from build123d import *

# Parameters (mm, degrees)
ESQUISSE1_R             = 1.5
BOSS_EXTRU_1_DEPTH      = 6
ESQUISSE2_R             = 1.5
ENL_V_MAT_EXTRU_1_DEPTH = 28.676885663
ESQUISSE3_R             = 1.5
ENL_V_MAT_EXTRU_2_DEPTH = 22.90010149


with BuildPart() as part:
    # Esquisse1 → Boss.-Extru.1 (new body)
    with BuildSketch(Plane.XY):
        with BuildLine():
            Line((-10, 4.424421769), (-10, -4.424421769))
            ThreePointArc((-10, -4.424421769), (-9.671289073, -5.165617412), (-8.901258038, -5.41953484))
            ThreePointArc((-8.901258038, -5.41953484), (-6.517555279, -6.205559881), (-5.5, -8.5))
            Line((-5.5, -8.5), (-5.5, -11.715481211))
            ThreePointArc((-5.5, -11.715481211), (-5.324186186, -12.281800142), (-4.858565737, -12.64898569))
            ThreePointArc((-4.858565737, -12.64898569), (0, -13.55), (4.858565737, -12.64898569))
            ThreePointArc((4.858565737, -12.64898569), (5.324186186, -12.281800142), (5.5, -11.715481211))
            Line((5.5, -11.715481211), (5.5, 1.096471453))
            ThreePointArc((5.5, 1.096471453), (5.66862168, 1.65217829), (6.117620177, 2.020476687))
            ThreePointArc((6.117620177, 2.020476687), (8.124885753, 5.023493695), (6.117620177, 8.026510703))
            ThreePointArc((6.117620177, 8.026510703), (5.66862168, 8.394809099), (5.5, 8.950515936))
            Line((5.5, 8.950515936), (5.5, 11.715481211))
            ThreePointArc((5.5, 11.715481211), (5.324186186, 12.281800142), (4.858565737, 12.64898569))
            ThreePointArc((4.858565737, 12.64898569), (0, 13.55), (-4.858565737, 12.64898569))
            ThreePointArc((-4.858565737, 12.64898569), (-5.324186186, 12.281800142), (-5.5, 11.715481211))
            Line((-5.5, 11.715481211), (-5.5, 8.5))
            ThreePointArc((-5.5, 8.5), (-6.517555279, 6.205559881), (-8.901258038, 5.41953484))
            ThreePointArc((-8.901258038, 5.41953484), (-9.671289073, 5.165617412), (-10, 4.424421769))
        make_face()
        with Locations((-4.874885753, -5.023493695)):
            Circle(ESQUISSE1_R, mode=Mode.SUBTRACT)
        with Locations((4.874885753, 5.023493695)):
            Circle(ESQUISSE1_R, mode=Mode.SUBTRACT)
        with BuildLine():
            Line((-3.5, 11.55), (3.5, 11.55))
            Line((3.5, 11.55), (3.5, 8.5))
            ThreePointArc((3.5, 8.5), (0, 5), (-3.5, 8.5))
            Line((-3.5, 8.5), (-3.5, 11.55))
        make_face(mode=Mode.SUBTRACT)
        with BuildLine():
            Line((-3.5, -11.55), (3.5, -11.55))
            Line((3.5, -11.55), (3.5, -8.5))
            ThreePointArc((3.5, -8.5), (0, -5), (-3.5, -8.5))
            Line((-3.5, -8.5), (-3.5, -11.55))
        make_face(mode=Mode.SUBTRACT)
        with BuildLine():
            Line((0, -3), (-8, -3))
            Line((-8, -3), (-8, 3))
            Line((-8, 3), (0, 3))
            ThreePointArc((0, 3), (3, 0), (0, -3))
        make_face(mode=Mode.SUBTRACT)
    extrude(amount=BOSS_EXTRU_1_DEPTH)

    # Esquisse2 → Enlèv. mat.-Extru.1 (cut, through all)
    with BuildSketch(Plane.XZ.offset(-11.55)):
        with Locations(Location((0, 3, 0), (0, 0, 270))):
            Circle(ESQUISSE2_R)
    enl_v_mat_extru_1 = extrude(amount=-ENL_V_MAT_EXTRU_1_DEPTH, mode=Mode.SUBTRACT)

    # Symétrie1: Enlèv. mat.-Extru.1 across plane
    add(enl_v_mat_extru_1.mirror(Plane.ZX), mode=Mode.SUBTRACT)

    # Esquisse3 → Enlèv. mat.-Extru.2 (cut, through all)
    with BuildSketch(Plane(origin=(-8, 0, 0), x_dir=(0, 0, -1), z_dir=(1, 0, 0))):
        with Locations((-3, 0)):
            Circle(ESQUISSE3_R)
    extrude(amount=-ENL_V_MAT_EXTRU_2_DEPTH, mode=Mode.SUBTRACT)


solid = part.part
For this review, take the finished solid that the model builds, in its own axes (mm). A direction names the side the tool comes from. Give positions to 0.01 mm unless a question says otherwise; leave off trailing zeros. Order: outer loops, then holes, each group sorted by start corner. A loop starts at its lowest first (then second) coordinate and runs counter-clockwise, first axis right, second up. Notation, with made-up numbers: (17.5, 2) - (64.5, 2) arc R25 ccw to (64.5, 38) - close; hole circle Ø9 at (87.25, -14.5). An arc over 180 degrees is marked (long way). Answer as a JSON object with one key per item and string values. Group by question number.
Item 1: Take a section at C-C on x = -2. Give the boundary of the cut face in (y, z).
Item 2: Wall thickness on line 1 along Y through (x, z) = (0, 2.5); line 2 along Y through (x, z) = (-5.25, 0.5); line 3 along Z through (x, y) = (0, -12.6): over which ranges is each line inside the solid? List them lowest first.
Item 3: Take a section at A-A on y = 0. Give the boundary of the cut face in (x, z).
Item 4: Take a section at D-D on x = -7.5. Give the boundary of the cut face in (y, z).
Item 5: Take a section at B-B on x = -4.25. Give the boundary of the cut face in (y, z).
Item 6: Machinability: for faces 4 (the flat face through (5.5, 10, 3)), 5 (the cylindrical face through (-8.99, 0.45, 1.57)), 6 (the flat face through (3.5, -10, 3)), 7 (the flat face through (-5.5, 10, 3)), which of the approach directions +Z, -Z, +X, -X, +Y, -Y give a long, thin tool a straight path to every point of the face, cutting with its end or side? Answer none if there is none.
Item 7: Draft analysis for pull direction X (two halves, no side actions). For faces 1 (the flat face through (-3.5, -10, 3)), 2 (the cylindrical face through (1.17, 13.5, 1.62)), 3 (the flat face through (-5.5, -10, 3)), state which applies: pulls with the +X half, pulls with the -X half, needs draft (parallel to the pull), parting line crosses it, or undercut.
Item 8: Clearance check with flat-ended pins moving along their axes: pin 1 Ø2.5 at (y, z) = (0, 3) entering from +X; pin 2 Ø2.5 at (x, y) = (-4.87, -5.02) entering from +Z; pin 3 Ø3.5 at (y, z) = (-9.5, 1.5) entering from -X; pin 4 Ø2.5 at (x, z) = (0, 3) entering from -Y. State where each tip first meets the part, or that it passes through.
Reported:
{
 "1": {"outline": "(-13.4, 0) - (-11.55, 0) - (-11.55, 6) - (-13.4, 6) - close; (-5.63, 0) - (-3, 0) - (-3, 6) - (-5.63, 6) - close; (3, 0) - (5.63, 0) - (5.63, 6) - (3, 6) - close; (11.55, 0) - (13.4, 0) - (13.4, 6) - (11.55, 6) - close"},
 "2": {"line 1": "-5 to -3, 3 to 5", "line 2": "-12.38 to -6.48, -3.57 to -3, 3 to 12.38", "line 3": "0 to 1.5, 4.5 to 6"},
 "3": {"outline": "(-10, 0) - (-8, 0) - (-8, 1.5) - (-10, 1.5) - close; (-10, 4.5) - (-8, 4.5) - (-8, 6) - (-10, 6) - close; (3, 0) - (5.5, 0) - (5.5, 6) - (3, 6) - close"},
 "4": {"outline": "(-5.6, 0) - (-3, 0) - (-3, 6) - (-5.6, 6) - close; (3, 0) - (5.6, 0) - (5.6, 6) - (3, 6) - close"},
 "5": {"outline": "(-12.87, 0) - (-6.39, 0) - (-6.39, 6) - (-12.87, 6) - close; (-3.66, 0) - (-3, 0) - (-3, 6) - (-3.66, 6) - close; (3, 0) - (12.87, 0) - (12.87, 6) - (3, 6) - close"},
 "6": {"face 4": "+Z, -Z, +X, +Y", "face 5": "-X", "face 6": "+Z, -Z", "face 7": "+Z, -Z, -X, +Y"},
 "7": {"face 1": "undercut", "face 2": "parting line crosses it", "face 3": "pulls with the -X half"},
 "8": {"pin 1": "x = 5.51", "pin 2": "through", "pin 3": "x = -5.59", "pin 4": "y = -5.23"}
}
